from build123d import *

# Parameters (mm, degrees)
SKETCH1_R           = 1
SKETCH1_R_2         = 2.25
SKETCH1_R_3         = 0.998074624
BOSS_EXTRUDE1_DEPTH = 1


with BuildPart() as part:
    # Sketch1 → Boss-Extrude1 (new body)
    with BuildSketch(Plane.XY):
        with BuildLine():
            Line((2.730147947, 1), (1.25, 1.108078099))
            ThreePointArc((1.25, 1.108078099), (-0.000138167, 0.017440541), (1.25, -1.073197017))
            Line((1.25, -1.073197017), (2.730147947, -1))
            ThreePointArc((2.730147947, -1), (2.918738623, -1.941142838), (3.225985726, -2.850491783))
            Line((3.225985726, -2.850491783), (1.890100953, -3.496967377))
            ThreePointArc((1.890100953, -3.496967377), (1.352768321, -5.066556292), (2.980738511, -5.38600704))
            Line((2.980738511, -5.38600704), (4.225985726, -4.582542591))
            ThreePointArc((4.225985726, -4.582542591), (4.656981948, -5.092323385), (5.131600413, -5.561760829))
            Line((5.131600413, -5.561760829), (7.44171219, -13.199988708))
            ThreePointArc((7.44171219, -13.199988708), (7.439945119, -13.784749424), (7.111476001, -14.268543034))
            ThreePointArc((7.111476001, -14.268543034), (5.923924571, -18.62818009), (9.697794763, -21.113057841))
            ThreePointArc((9.697794763, -21.113057841), (10.380528535, -21.341854349), (10.732574986, -21.969975788))
            ThreePointArc((10.732574986, -21.969975788), (10.791766979, -22.393908793), (10.847713449, -22.818282305))
            ThreePointArc((10.847713449, -22.818282305), (11.790244876, -24.335347863), (11.16321594, -26.007678007))
            ThreePointArc((11.16321594, -26.007678007), (10.570290463, -27.483765064), (11.290805177, -28.901951288))
            ThreePointArc((11.290805177, -28.901951288), (11.931562756, -30.214937196), (11.277042334, -31.52111685))
            ThreePointArc((11.277042334, -31.52111685), (10.500432467, -32.761716535), (11.145287395, -34.075631519))
            ThreePointArc((11.145287395, -34.075631519), (11.711049486, -35.240414102), (10.937199745, -36.278663489))
            ThreePointArc((10.937199745, -36.278663489), (10.185540032, -37.265502357), (10.650830557, -38.415436269))
            ThreePointArc((10.650830557, -38.415436269), (11.153884573, -39.735845823), (10.230304321, -40.805212107))
            ThreePointArc((10.230304321, -40.805212107), (9.263580844, -41.700908083), (9.768401259, -42.918274877))
            ThreePointArc((9.768401259, -42.918274877), (10.29278617, -44.215864041), (9.202326649, -45.093141196))
            ThreePointArc((9.202326649, -45.093141196), (8.144843355, -45.909982105), (8.571180325, -47.176369398))
            ThreePointArc((8.571180325, -47.176369398), (8.845608938, -48.309992252), (7.932024848, -49.035096348))
            ThreePointArc((7.932024848, -49.035096348), (7.054134874, -49.652663659), (7.297145805, -50.698142438))
            ThreePointArc((7.297145805, -50.698142438), (7.486031135, -51.627523472), (6.693279806, -52.148073283))
            ThreePointArc((6.693279806, -52.148073283), (5.736341709, -52.667939714), (5.979078831, -53.729575393))
            ThreePointArc((5.979078831, -53.729575393), (6.146574337, -54.831276595), (5.172832259, -55.373149872))
            ThreePointArc((5.172832259, -55.373149872), (4.397991341, -55.805643097), (4.477975588, -56.689402883))
            ThreePointArc((4.477975588, -56.689402883), (4.477842946, -57.805544451), (3.519463877, -58.377629741))
            ThreePointArc((3.519463877, -58.377629741), (2.763689302, -58.882818754), (2.639049746, -59.78330536))
            ThreePointArc((2.639049746, -59.78330536), (2.762025793, -60.669472955), (2.167842085, -61.338324084))
            ThreePointArc((2.167842085, -61.338324084), (1.802507902, -61.611764905), (1.596700522, -62.019051378))
            ThreePointArc((1.596700522, -62.019051378), (1.419841706, -62.882777694), (1.305095034, -63.756926075))
            ThreePointArc((1.305095034, -63.756926075), (1.556005476, -64.519090759), (2.286327304, -64.851477705))
            Line((2.286327304, -64.851477705), (4.151796088, -64.878115588))
            ThreePointArc((4.151796088, -64.878115588), (4.56955608, -64.79320511), (4.913989999, -64.54201101))
            Line((4.913989999, -64.54201101), (19.858030846, -47.704114694))
            ThreePointArc((19.858030846, -47.704114694), (21.299586827, -45.585122466), (22.155211357, -43.169316519))
            Line((22.155211357, -43.169316519), (25.087470282, -29.538838187))
            ThreePointArc((25.087470282, -29.538838187), (25.281255234, -26.663292069), (24.646889926, -23.851904734))
            Line((24.646889926, -23.851904734), (16.818242905, -3.45834767))
            ThreePointArc((16.818242905, -3.45834767), (17.313669941, -2.262858102), (17.596216694, -1))
            Line((17.596216694, -1), (19.076364641, -1.108078099))
            ThreePointArc((19.076364641, -1.108078099), (20.326502808, -0.017440541), (19.076364641, 1.073197017))
            Line((19.076364641, 1.073197017), (17.596216694, 1))
            ThreePointArc((17.596216694, 1), (17.407626018, 1.941142838), (17.100378915, 2.850491783))
            Line((17.100378915, 2.850491783), (18.436263688, 3.496967377))
            ThreePointArc((18.436263688, 3.496967377), (18.97359632, 5.066556292), (17.34562613, 5.38600704))
            Line((17.34562613, 5.38600704), (16.100378915, 4.582542591))
            ThreePointArc((16.100378915, 4.582542591), (15.466483179, 5.303300859), (14.745724911, 5.937196595))
            Line((14.745724911, 5.937196595), (15.579397264, 7.165003268))
            ThreePointArc((15.579397264, 7.165003268), (15.259946516, 8.792973458), (13.690357601, 8.255640826))
            Line((13.690357601, 8.255640826), (13.013674103, 6.937196595))
            ThreePointArc((13.013674103, 6.937196595), (12.104325159, 7.244443697), (11.16318232, 7.433034374))
            Line((11.16318232, 7.433034374), (11.27126042, 8.91318232))
            ThreePointArc((11.27126042, 8.91318232), (10.180622862, 10.163320487), (9.089985304, 8.91318232))
            Line((9.089985304, 8.91318232), (9.16318232, 7.433034374))
            ThreePointArc((9.16318232, 7.433034374), (8.222039482, 7.244443697), (7.312690537, 6.937196595))
            Line((7.312690537, 6.937196595), (6.666214944, 8.273081368))
            ThreePointArc((6.666214944, 8.273081368), (5.096626029, 8.810413999), (4.77717528, 7.18244381))
            Line((4.77717528, 7.18244381), (5.58063973, 5.937196595))
            ThreePointArc((5.58063973, 5.937196595), (4.859881461, 5.303300859), (4.225985726, 4.582542591))
            Line((4.225985726, 4.582542591), (2.998179052, 5.416214944))
            ThreePointArc((2.998179052, 5.416214944), (1.370208862, 5.096764195), (1.907541494, 3.52717528))
            Line((1.907541494, 3.52717528), (3.225985726, 2.850491783))
            ThreePointArc((3.225985726, 2.850491783), (2.918738623, 1.941142838), (2.730147947, 1))
        make_face()
        with Locations((10.16318232, 0)):
            Circle(SKETCH1_R, mode=Mode.SUBTRACT)
        with Locations((15.627966379, -9.260281964)):
            Circle(SKETCH1_R_2, mode=Mode.SUBTRACT)
        with Locations((9.121782476, -17.526259213)):
            Circle(SKETCH1_R_3, mode=Mode.SUBTRACT)
        with Locations((22, -26.49969455)):
            Circle(SKETCH1_R, mode=Mode.SUBTRACT)
        with Locations((21.500000045, -33.166361217)):
            Circle(SKETCH1_R, mode=Mode.SUBTRACT)
        with Locations((18.474150388, -39.833027883)):
            Circle(SKETCH1_R, mode=Mode.SUBTRACT)
        with Locations((17.55481685, -46.49969455)):
            Circle(SKETCH1_R, mode=Mode.SUBTRACT)
        with BuildLine():
            Line((14.500290742, -21.375988683), (12.638736062, -16.487053928))
            ThreePointArc((12.638736062, -16.487053928), (13.337027802, -14.929994394), (14.894087335, -15.628286133))
            Line((14.894087335, -15.628286133), (16.755642015, -20.517220889))
            ThreePointArc((16.755642015, -20.517220889), (16.057350276, -22.074280422), (14.500290742, -21.375988683))
        make_face(mode=Mode.SUBTRACT)
    extrude(amount=BOSS_EXTRUDE1_DEPTH)


solid = part.part
The model under review builds one solid part; all positions refer to its coordinate system, in mm. A direction names the side the tool comes from. Round coordinates to 2 decimals unless told otherwise and drop trailing zeros. Loops run counter-clockwise (first coordinate to the right, second up) from the corner with the lowest first, then second, coordinate; pieces in that order, holes last. Notation, with made-up numbers: (31, -2) -> (45, -2) arc R18 cw to (45, 4) -> close; hole circle Ø2 at (-0.75, 18.5). An arc over 180 degrees is marked (long way). Write item = value, one per line. Start each with the question number.
Item 1: Mouldability with a two-part tool opening along Y and no side actions: class faces 1 (the flat face through (12, -27, 0)), 2 (the cylindrical face through (21.28, -45.62, 0.49)), 3 (the flat face through (6.27, -9.33, 0.49)) as released by +Y, released by -Y, zero draft, split by the parting line, or undercut.
Item 2: Take a section at A-A on y = 0. Give the boundary of the cut face in (x, z), plus the area to 3 significant figures.
Item 3: For faces 4 (the flat face through (13.583, -18.966, 0.493)), 5 (the flat face through (20.79, -13.8, 0.49)), 6 (the flat face through (12.28, -56.24, 0.49)), list the 3-axis set-ups (+Z, -Z, +X, -X, +Y, -Y) from which the entire face can be reached by the end or side of a thin tool; tool diameter is ignored.
Item 4: Insertion check: pin 1 (3.5 mm diameter, centred on x = 15.63, y = -9.26, fed in from -Z). The pin has a flat end and moves straight along its axis. Give the tip position at first contact, or say it passes through.
Item 5: Take a section at B-B on z = 0.25. Count the separate pieces of the cut face and the enclosed holes in it, plus the area to 3 significant figures.
Item 6: To check wall thickness, follow L1, parallel to Y at x = 2, z = 0.65; L2, parallel to Y at x = 11.5, z = 0.9; L3, parallel to Y at x = 5, z = 0.6. State the ranges of each line that lie inside material, in increasing order.
Result:
q1.face_1 = zero draft
q1.face_2 = released by -Y
q1.face_3 = undercut
q2.outline = (0, 0) -> (9.16, 0) -> (9.16, 1) -> (0, 1) -> close; (11.16, 0) -> (20.33, 0) -> (20.33, 1) -> (11.16, 1) -> close
q2.area = 18.3 mm²
q3.face_4 = +Z, -Z
q3.face_5 = +Z, -Z, +X
q3.face_6 = +Z, -Z, +X, -Y
q4.pin_1 = through
q5.separate_pieces = 1
q5.enclosed_holes = 8
q5.area = 852 mm²
q6.L1 = -64.81 to -61.43, -5.57 to -3.44, -1.04 to 1.05, 3.48 to 5.6
q6.L2 = -57.12 to -35.83, -34.42 to -31.32, -29.09 to -25.59, -23.47 to 7.38
q6.L3 = -64.45 to -55.38, -5.44 to 5.44, 6.84 to 8.75
